For this review, take the finished solid that the model builds, in its own axes (mm). Face numbers are marked on the shaded views. A direction names the side the tool comes from. Give positions to 0.01 mm unless a question says otherwise; leave off trailing zeros. Loops run counter-clockwise (first coordinate to the right, second up) from the corner with the lowest first, then second, coordinate; pieces in that order, holes last. Notation, with made-up numbers: (-33, 19.5) -> (-29, 19.5) arc R24 cw to (-29, 44.5) -> close; hole circle Ø8 at (80, 89.25). An arc over 180 degrees is marked (long way). Answer as CSV lines item,"result". Start each with the question number.
Item 1: Add section B-B on z = -1. State the section outline as (x, y) points, plus the area to 3 significant figures.
Item 2: Add section A-A on y = 0. State the section outline as (x, z) points.
Item 3: Add section C-C on z = 2. State the section outline as (x, y) points.
Item 4: Machinability: for the marked faces 4 and 5, which of the approach directions +Z, -Z, +X, -X, +Y, -Y give a long, thin tool a straight path to every point of the face, cutting with its end or side? Answer none if there is none.
Item 5: The part is to be moulded in two halves that separate along X. For the marked faces 1, 2 and 3, say which applies: +X half, -X half, draft (parallel to the pull), parting line (faces both ways), or undercut.
Item 6: For L1, parallel to Y at x = -0.75, z = 3; L2, parallel to Y at x = -1.5, z = 1.75; L3, parallel to X at y = 0, z = 0, list the stretches that pass through material, from the lowest coordinate up. Write a range as from..to.
Item 7: Clearance check with flat-ended pins moving along their axes: P1, Ø0.8, axis at x = 0.5, y = 0.5, coming from the +Z side; P2, Ø1.2, axis at y = 0, z = 3, coming from the -X side; P3, Ø2, axis at x = 1, z = -3, coming from the +Y side. State where each tip first meets the part, or that it passes through.
```python
from build123d import *

# Parameters (mm, degrees)
SKETCH3_W          = 8
SKETCH3_H          = 2
CHAMFER1_SIZE      = 0.6
CUT_EXTRUDE1_DEPTH = 1.61
SKETCH9_R          = 1.443375673
CUT_EXTRUDE2_DEPTH = 1.61
CUT_EXTRUDE2_DRAFT = -45


with BuildPart() as part:
    # Sketch3 → Revolve1 (revolve)
    with BuildSketch(Plane(origin=(0, 0, 0), x_dir=(0, 0, -1), z_dir=(1, 0, 0))):
        with Locations((0, 1)):
            Rectangle(SKETCH3_W, SKETCH3_H)
    revolve(axis=Axis((0, 0, -4), (0, 0, 1)))

    # Chamfer1
    chamfer1_edges = [part.edges().sort_by_distance(p)[0] for p in [
        (0, -2, -4),
    ]]
    chamfer(chamfer1_edges, length=CHAMFER1_SIZE)

    # Sketch6 → Revolve2 (revolve)
    with BuildSketch(Plane(origin=(0, 0, 0), x_dir=(0, 0, -1), z_dir=(1, 0, 0))):
        Polygon((-4, 4), (-3.7, 4), (-1.7, 2), (-1.7, 0), (-4, 0), align=None)
    revolve(axis=Axis((0, 0, -4), (0, 0, 1)))

    # Sketch8 → Cut-Extrude1 (cut)
    with BuildSketch(Plane.XY.offset(4)):
        Polygon((0, 1.443375673), (-1.25, 0.721687836), (-1.25, -0.721687836), (0, -1.443375673), (1.25, -0.721687836), (1.25, 0.721687836), align=None)
    extrude(amount=-CUT_EXTRUDE1_DEPTH, mode=Mode.SUBTRACT)


with BuildPart() as cut_extrude2_tool:
    # Sketch9 → Cut-Extrude2 (with draft: the straight prism first)
    with BuildSketch(Plane.XY.offset(4)):
        Circle(SKETCH9_R)
    extrude(amount=-CUT_EXTRUDE2_DEPTH)
    # Cut-Extrude2: the draft: its side faces are tilted about the plane it starts from
    cut_extrude2_sides = [cut_extrude2_tool.faces().sort_by_distance(p)[0] for p in [
        (-1.443375673, 0, 3.195),
    ]]
    draft(cut_extrude2_sides, Plane.XY.offset(4), CUT_EXTRUDE2_DRAFT)


with BuildPart() as part_1:
    add(part.part)

    # Cut-Extrude2: cut by cut_extrude2_tool
    add(cut_extrude2_tool.part, mode=Mode.SUBTRACT)


solid = part_1.part
```
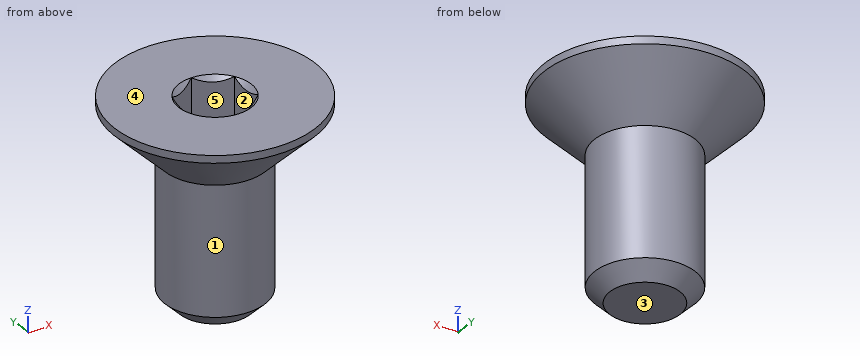
Computed values:
1,outline,"circle Ø4 at (0, 0)"
1,area,"12.6 mm²"
2,outline,"(-4, 3.7) -> (-2, 1.7) -> (-2, -3.4) -> (-1.4, -4) -> (1.4, -4) -> (2, -3.4) -> (2, 1.7) -> (4, 3.7) -> (4, 4) -> (1.44, 4) -> (1.25, 3.81) -> (1.25, 2.39) -> (-1.25, 2.39) -> (-1.25, 3.81) -> (-1.44, 4) -> (-4, 4) -> close"
3,outline,"circle Ø4.6 at (0, 0)"
4,face 4,"+Z, +X, -X, +Y, -Y"
4,face 5,"+Z"
5,face 1,"parting line"
5,face 2,"undercut"
5,face 3,"draft"
6,L1,"-3.21..-1.01, 1.01..3.21"
6,L2,"-1.4..1.4"
6,L3,"-2..2"
7,P1,"z = 2.39"
7,P2,"x = -3.9"
7,P3,"y = 2"
